Could you check a few things on this model? Use its own coordinates, in mm. A direction names the side the tool comes from. Round coordinates to 2 decimals unless told otherwise and drop trailing zeros. Order: outer loops, then holes, each group sorted by start corner. A loop starts at its lowest first (then second) coordinate and runs counter-clockwise, first axis right, second up. Notation, with made-up numbers: (-15, -1.5) - (35, -1.5) arc R9 cw to (35, 10.5) - close; hole circle Ø5 at (-26.75, 23). An arc over 180 degrees is marked (long way). Use one line per item in the form item = value.
from build123d import *

# Parameters (mm, degrees)
SKETCH1_R           = 2.75
BOSS_EXTRUDE2_DEPTH = 2


with BuildPart() as part:
    # Sketch1 → Boss-Extrude2 (new body)
    with BuildSketch(Plane.XY):
        with BuildLine():
            Line((35, 0), (45, 0))
            ThreePointArc((45, 0), (49, 4), (45, 8))
            Line((45, 8), (0, 8))
            ThreePointArc((0, 8), (-4, 4), (0, 0))
            Line((0, 0), (27, 0))
            Line((27, 0), (27, -15))
            ThreePointArc((27, -15), (31, -19), (35, -15))
            Line((35, -15), (35, 0))
        make_face()
        with Locations((45, 4)):
            Circle(SKETCH1_R, mode=Mode.SUBTRACT)
        with Locations((31, -15)):
            Circle(SKETCH1_R, mode=Mode.SUBTRACT)
    extrude(amount=BOSS_EXTRUDE2_DEPTH)


solid = part.part
Item 1: Imagine slicing it at C-C on x = 29. Please give me the cut outline in (y, z), plus the area to 3 significant figures.
Found:
outline = (-18.46, 0) - (-16.89, 0) - (-16.89, 2) - (-18.46, 2) - close; (-13.11, 0) - (8, 0) - (8, 2) - (-13.11, 2) - close
area = 45.4 mm2
Item 2: For faces 1 (the face through (13, 0, 1)), 2 (the face through (22, 1, 2)), 3 (the face through (35, -8, 1)), which set-ups out of +Z, -Z, +X, -X, +Y, -Y let a thin tool reach every point of the face, with its end or its side?
Found:
face_1 = +Z, -Z, -X, -Y
face_2 = +Z, +X, -X, +Y, -Y
face_3 = +Z, -Z, +X, -Y
Item 3: I need wall thicknesses on L1, parallel to Y at x = 45, z = 0.8; L2, parallel to Y at x = 31, z = 0.7; L3, parallel to Y at x = 14, z = 1.2. Which ranges of each line are inside material? Lowest first, please.
Found:
L1 = 0 to 1.25, 6.75 to 8
L2 = -19 to -17.75, -12.25 to 8
L3 = 0 to 8
Item 4: If we mould it in two halves opening along X, with no side actions, what happens to faces 4 (the face through (42.253, 4.121, 0.986)), 5 (the face through (49, 4, 1)), 6 (the face through (27, -7, 1)), 7 (the face through (22, 1, 0))? For each: released by +X, released by -X, zero draft, split by the parting line, or undercut.
Found:
face_4 = undercut
face_5 = released by +X
face_6 = released by -X
face_7 = zero draft
Item 5: Imagine slicing it at B-B on z = 1.6. Please give me the cut outline in (x, y), plus the area to 3 significant figures.
Found:
outline = (0, 0) - (27, 0) - (27, -15) arc R4 ccw to (35, -15) - (35, 0) - (45, 0) arc R4 ccw to (45, 8) - (0, 8) arc R4 ccw to start; hole circle Ø5.5 at (31, -15); hole circle Ø5.5 at (45, 4)
area = 508 mm2
Item 6: Will these pins go through, and if not, where does the flat tip stop? P1, Ø3.5, axis at x = 45, y = 4, coming from the -Z side; P2, Ø1, axis at x = 16, z = 0.5, coming from the -Y side; P3, Ø0.6, axis at y = -5, z = 1.5, coming from the +X side.
Found:
P1 = through
P2 = 0
P3 = 35
Item 7: Imagine slicing it at A-A on y = 4. Please give me the cut outline in (x, z), plus the area to 3 significant figures.
Found:
outline = (-4, 0) - (42.25, 0) - (42.25, 2) - (-4, 2) - close; (47.75, 0) - (49, 0) - (49, 2) - (47.75, 2) - close
area = 95.0 mm2
Item 8: Imagine slicing it at D-D on y = -5.25. Please give me the cut outline in (x, z).
Found:
outline = (27, 0) - (35, 0) - (35, 2) - (27, 2) - close
